```python
from build123d import *

# Parameters (mm, degrees)
F0_R     = 14.2875
F1_DEPTH = 12.7
F2_DEPTH = 25.4


with BuildPart() as f1:
    # F0 (on Top) → F1 (new body)
    with BuildSketch(Plane.XY):
        with BuildLine():
            ThreePointArc((5.0426470588, -28.1265414802), (21.9160245563, -18.3362616868), (28.575, 0))
            ThreePointArc((28.575, 0), (21.9160245563, 18.3362616868), (5.0426470588, 28.1265414802))
            ThreePointArc((5.0426470588, 28.1265414802), (-28.575, 0), (5.0426470588, -28.1265414802))
        make_face()
        with BuildLine():
            ThreePointArc((-13.4703841816, 4.7625), (0, 14.2875), (13.4703841816, 4.7625))
            Line((13.4703841816, 4.7625), (19.05, 4.7625))
            Line((19.05, 4.7625), (19.05, -4.7625))
            Line((19.05, -4.7625), (13.4703841816, -4.7625))
            ThreePointArc((13.4703841816, -4.7625), (0, -14.2875), (-13.4703841816, -4.7625))
            Line((-13.4703841816, -4.7625), (-19.05, -4.7625))
            Line((-19.05, -4.7625), (-19.05, 4.7625))
            Line((-19.05, 4.7625), (-13.4703841816, 4.7625))
        make_face(mode=Mode.SUBTRACT)
        with BuildLine():
            ThreePointArc((73.025, 0), (68.5856830375, 12.2241744579), (57.3367647059, 18.7510276535))
            ThreePointArc((57.3367647059, 18.7510276535), (34.925, 0), (57.3367647059, -18.7510276535))
            ThreePointArc((57.3367647059, -18.7510276535), (68.5856830375, -12.2241744579), (73.025, 0))
        make_face()
        with Locations((53.975, 0)):
            Circle(F0_R, mode=Mode.SUBTRACT)
        with BuildLine():
            ThreePointArc((5.0426470588, 28.1265414802), (21.9160245563, 18.3362616868), (28.575, 0))
            ThreePointArc((28.575, 0), (21.9160245563, -18.3362616868), (5.0426470588, -28.1265414802))
            Line((5.0426470588, -28.1265414802), (57.3367647059, -18.7510276535))
            ThreePointArc((57.3367647059, -18.7510276535), (34.925, 0), (57.3367647059, 18.7510276535))
            Line((57.3367647059, 18.7510276535), (5.0426470588, 28.1265414802))
        make_face()
        with BuildLine():
            ThreePointArc((-13.4703841816, -4.7625), (-14.2875, 0), (-13.4703841816, 4.7625))
            Line((-13.4703841816, 4.7625), (-19.05, 4.7625))
            Line((-19.05, 4.7625), (-19.05, -4.7625))
            Line((-19.05, -4.7625), (-13.4703841816, -4.7625))
        make_face()
    extrude(amount=F1_DEPTH)

    # F0 (on Top) → F2 (join)
    with BuildSketch(Plane.XY):
        with BuildLine():
            ThreePointArc((5.0426470588, -28.1265414802), (21.9160245563, -18.3362616868), (28.575, 0))
            ThreePointArc((28.575, 0), (21.9160245563, 18.3362616868), (5.0426470588, 28.1265414802))
            ThreePointArc((5.0426470588, 28.1265414802), (-28.575, 0), (5.0426470588, -28.1265414802))
        make_face()
        with BuildLine():
            ThreePointArc((-13.4703841816, 4.7625), (0, 14.2875), (13.4703841816, 4.7625))
            Line((13.4703841816, 4.7625), (19.05, 4.7625))
            Line((19.05, 4.7625), (19.05, -4.7625))
            Line((19.05, -4.7625), (13.4703841816, -4.7625))
            ThreePointArc((13.4703841816, -4.7625), (0, -14.2875), (-13.4703841816, -4.7625))
            Line((-13.4703841816, -4.7625), (-19.05, -4.7625))
            Line((-19.05, -4.7625), (-19.05, 4.7625))
            Line((-19.05, 4.7625), (-13.4703841816, 4.7625))
        make_face(mode=Mode.SUBTRACT)
        with BuildLine():
            ThreePointArc((-13.4703841816, -4.7625), (-14.2875, 0), (-13.4703841816, 4.7625))
            Line((-13.4703841816, 4.7625), (-19.05, 4.7625))
            Line((-19.05, 4.7625), (-19.05, -4.7625))
            Line((-19.05, -4.7625), (-13.4703841816, -4.7625))
        make_face()
    extrude(amount=F2_DEPTH)


solid = f1.part
```
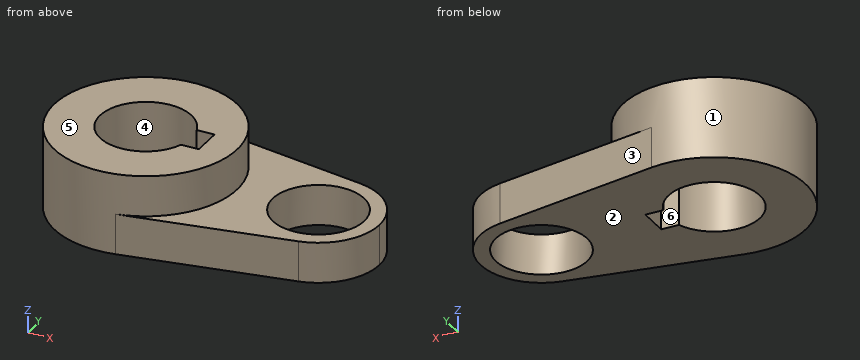
Check sheet for the modelled part. Datum: model origin and axes. Units: mm. Face numbers are marked on the shaded views. A direction names the side the tool comes from. Round coordinates to 2 decimals unless told otherwise and drop trailing zeros. Order: outer loops, then holes, each group sorted by start corner. A loop starts at its lowest first (then second) coordinate and runs counter-clockwise, first axis right, second up. Notation, with made-up numbers: (63.5, 27.5) - (79.5, 27.5) arc R22 ccw to (79.5, 49.5) - close; hole circle Ø5 at (55, -17). An arc over 180 degrees is marked (long way). Answer as CSV lines item,"result". Start each with the question number.
1) Draft check along Y on the marked faces 1, 2, 3 and 4. Enter one of: +Y half, -Y half, draft (parallel to the pull), parting line (faces both ways), or undercut.
2) Section check B-B (y = -2). Record the cut outline in (x, z), then the cut area to 3 significant figures.
3) Section check A-A (z = 4.25). Give the number of separate pieces and of enclosed holes in the cut face, then the cut area to 3 significant figures.
4) Section check C-C (x = 0). Record the cut outline in (y, z) (1 decimal), then the cut area to 3 significant figures.
5) Depth check by flat-ended pin: pin 1 (2 mm diameter, centred on y = -17.5, z = 16.5, fed in from +X); pin 2 (8 mm diameter, centred on y = -3.5, z = 14, fed in from -X) (3 decimals); pin 3 (10 mm diameter, centred on x = 44, y = 17, fed in from +Z). Enter the tip coordinate at first touch or a pass-through.
6) Tool access check on the marked faces 5 and 6. Record the directions out of +Z, -Z, +X, -X, +Y, -Y that give a thin tool (end or side, any length) a straight path to the whole face; none if there is none.
7) Scan lines: probe 1 along X at (y, z) = (-6.5, 7); probe 2 along X at (y, z) = (7, 7); probe 3 along Z at (x, y) = (36.5, -2.5). Record each from-to range of solid material in increasing order.
8) Section check D-D (y = -8). Record the cut outline in (x, z).
Determined:
1,face 1,"parting line"
1,face 2,"draft"
1,face 3,"+Y half"
1,face 4,"undercut"
2,outline,"(-28.5, 0) - (-14.15, 0) - (-14.15, 25.4) - (-28.5, 25.4) - close; (19.05, 0) - (39.83, 0) - (39.83, 12.7) - (28.5, 12.7) - (28.5, 25.4) - (19.05, 25.4) - close; (68.12, 0) - (72.92, 0) - (72.92, 12.7) - (68.12, 12.7) - close"
2,area,"810 mm^2"
3,separate pieces,"1"
3,enclosed holes,"2"
3,area,"3,130 mm^2"
4,outline,"(-28.6, 0) - (-14.3, 0) - (-14.3, 25.4) - (-28.6, 25.4) - close; (14.3, 0) - (28.6, 0) - (28.6, 25.4) - (14.3, 25.4) - close"
4,area,"726 mm^2"
5,pin 1,"x = 23.33"
5,pin 2,"x = -28.575"
5,pin 3,"z = 12.7"
6,face 5,"+Z, +X, -X, +Y, -Y"
6,face 6,"+Z, -Z"
7,probe 1,"-27.83 to -12.72, 12.72 to 41.25, 66.7 to 71.88"
7,probe 2,"-27.7 to -12.46, 12.46 to 41.52, 66.43 to 71.69"
7,probe 3,"0 to 12.7"
8,outline,"(-27.43, 0) - (-11.84, 0) - (-11.84, 25.4) - (-27.43, 25.4) - close; (11.84, 0) - (42.14, 0) - (42.14, 12.7) - (27.43, 12.7) - (27.43, 25.4) - (11.84, 25.4) - close; (65.81, 0) - (71.26, 0) - (71.26, 12.7) - (65.81, 12.7) - close"
